from build123d import *

# Parameters (mm, degrees)
SKETCH2_W           = 120
SKETCH2_H           = 100
SKETCH2_R           = 10
BOSS_EXTRUDE1_DEPTH = 20


with BuildPart() as part:
    # Sketch2 → Boss-Extrude1 (new body)
    with BuildSketch(Plane.XY):
        Rectangle(SKETCH2_W, SKETCH2_H)
        with Locations((-40, -30)):
            Circle(SKETCH2_R, mode=Mode.SUBTRACT)
        with Locations(Location((40, -30, 0), (0, 0, 180))):
            Circle(SKETCH2_R, mode=Mode.SUBTRACT)
        with Locations((40, 30)):
            Circle(SKETCH2_R, mode=Mode.SUBTRACT)
        with Locations(Location((-40, 30, 0), (0, 0, 180))):
            Circle(SKETCH2_R, mode=Mode.SUBTRACT)
        with BuildLine():
            Line((-30, 10), (30, 10))
            ThreePointArc((30, 10), (40, 0), (30, -10))
            Line((30, -10), (-30, -10))
            ThreePointArc((-30, -10), (-40, 0), (-30, 10))
        make_face(mode=Mode.SUBTRACT)
    extrude(amount=BOSS_EXTRUDE1_DEPTH)


solid = part.part
Could you check a few things on this model? Use its own coordinates, in mm. A direction names the side the tool comes from. Give positions to 0.01 mm unless a question says otherwise; leave off trailing zeros. Order: outer loops, then holes, each group sorted by start corner. A loop starts at its lowest first (then second) coordinate and runs counter-clockwise, first axis right, second up. Notation, with made-up numbers: (10.25, -13) -> (60.25, -13) arc R16 ccw to (60.25, 11) -> close; hole circle Ø6 at (68, -16). An arc over 180 degrees is marked (long way). Answer in a Markdown table with one row per item. Add a question column.
Item 1: Imagine slicing it at A-A (y = 30). List the corners of the cut face in (x, z) for me.
Item 2: Please list where these lines run through material, in increasing order: probe 1 along Y at (x, z) = (-49, 6); probe 2 along Y at (x, z) = (13, 8.25); probe 3 along X at (y, z) = (22.5, 12.5).
Item 3: Imagine slicing it at D-D (y = 4). List the corners of the cut face in (x, z) for me.
Item 4: Imagine slicing it at C-C (x = -46). List the corners of the cut face in (y, z) for me.
Item 5: We'd pull the mould along Y, two halves only. Please class faces 1 (the cylindrical face through (42.17, -20.24, 9.86)), 2 (the flat face through (-1, 12, 0)), 3 (the flat face through (-1, 50, 10)): pulls with the +Y half, pulls with the -Y half, needs draft (parallel to the pull), parting line crosses it, or undercut.
Item 6: For faces 4 (the flat face through (0, 10, 10)), 5 (the flat face through (-1, -50, 10)), which set-ups out of +Z, -Z, +X, -X, +Y, -Y let a thin tool reach every point of the face, with its end or its side?
Item 7: I'm going to push a flat-ended pin straight in: P1, Ø12, axis at x = -40, y = -30, coming from the -Z side. Where does the tip first touch, or does it pass through?
Item 8: Imagine slicing it at B-B (x = 10). List the corners of the cut face in (y, z) for me.
Result:
| question | item | result |
|---|---|---|
| 1 | outline | (-60, 0) -> (-50, 0) -> (-50, 20) -> (-60, 20) -> close; (-30, 0) -> (30, 0) -> (30, 20) -> (-30, 20) -> close; (50, 0) -> (60, 0) -> (60, 20) -> (50, 20) -> close |
| 2 | probe 1 | -50 to -34.36, -25.64 to 25.64, 34.36 to 50 |
| 2 | probe 2 | -50 to -10, 10 to 50 |
| 2 | probe 3 | -60 to -46.61, -33.39 to 33.39, 46.61 to 60 |
| 3 | outline | (-60, 0) -> (-39.17, 0) -> (-39.17, 20) -> (-60, 20) -> close; (39.17, 0) -> (60, 0) -> (60, 20) -> (39.17, 20) -> close |
| 4 | outline | (-50, 0) -> (-38, 0) -> (-38, 20) -> (-50, 20) -> close; (-22, 0) -> (22, 0) -> (22, 20) -> (-22, 20) -> close; (38, 0) -> (50, 0) -> (50, 20) -> (38, 20) -> close |
| 5 | face 1 | undercut |
| 5 | face 2 | needs draft |
| 5 | face 3 | pulls with the +Y half |
| 6 | face 4 | +Z, -Z |
| 6 | face 5 | +Z, -Z, +X, -X, -Y |
| 7 | P1 | through |
| 8 | outline | (-50, 0) -> (-10, 0) -> (-10, 20) -> (-50, 20) -> close; (10, 0) -> (50, 0) -> (50, 20) -> (10, 20) -> close |
